Part model, mm, in its own coordinate system. Face numbers are marked on the shaded views. A direction names the side the tool comes from. Round coordinates to 2 decimals unless told otherwise and drop trailing zeros. Order: outer loops, then holes, each group sorted by start corner. A loop starts at its lowest first (then second) coordinate and runs counter-clockwise, first axis right, second up. Notation, with made-up numbers: (-26.75, -31) -> (14.25, -31) arc R28 cw to (14.25, 7) -> close; hole circle Ø3 at (39.25, 54). An arc over 180 degrees is marked (long way). Return JSON: item names as keys, results as strings. Group by question number.
from build123d import *

# Parameters (mm, degrees)
ESQUISSE1_W             = 82.5
ESQUISSE1_H             = 16.543047786
BOSS_EXTRU_1_DEPTH      = 10
CONG_1_R                = 10
ESQUISSE2_W             = 5
ESQUISSE2_H             = 5
ENL_V_MAT_EXTRU_2_DEPTH = 21
ESQUISSE4_W             = 5
ESQUISSE4_H             = 5
ENL_V_MAT_EXTRU_3_DEPTH = 100
ESQUISSE5_R             = 5.960029696
ESQUISSE5_R_2           = 5.029757688
BOSS_EXTRU_4_DEPTH      = 80
ESQUISSE8_R             = 4.979256744
ENL_V_MAT_EXTRU_5_DEPTH = 80
ESQUISSE9_W             = 44.615478915
ESQUISSE9_H             = 9.98536909
BOSS_EXTRU_5_DEPTH      = 10
ESQUISSE10_W            = 10
ESQUISSE10_H            = 10
BOSS_EXTRU_6_DEPTH      = 5
ESQUISSE13_W            = 10
ESQUISSE13_H            = 5
BOSS_EXTRU_7_DEPTH      = 80
ESQUISSE15_R            = 4.979256744
ENL_V_MAT_EXTRU_6_DEPTH = 80


with BuildPart() as part:
    # Esquisse1 → Boss.-Extru.1 (new body)
    with BuildSketch(Plane(origin=(0, 0, 0), x_dir=(1, 0, 0), z_dir=(0, 1, 0))):
        with Locations((-15.683865756, -16.543047786)):
            Rectangle(ESQUISSE1_W, ESQUISSE1_H)
    extrude(amount=BOSS_EXTRU_1_DEPTH)

    # Congé1
    cong_1_edges = [part.edges().sort_by_distance(p)[0] for p in [
        (25.566134244, 5, 24.814571679),
        (-56.933865756, 5, 24.814571679),
    ]]
    fillet(cong_1_edges, radius=CONG_1_R)

    # Esquisse2 → Enlèv. mat.-Extru.2 (cut)
    with BuildSketch(Plane.XY.offset(24.814571679)):
        with Locations((-42.433865756, 5)):
            Rectangle(ESQUISSE2_W, ESQUISSE2_H)
    extrude(amount=-ENL_V_MAT_EXTRU_2_DEPTH, mode=Mode.SUBTRACT)

    # Esquisse4 → Enlèv. mat.-Extru.3 (cut)
    with BuildSketch(Plane.XY.offset(24.814571679)):
        with Locations((11.066134244, 5)):
            Rectangle(ESQUISSE4_W, ESQUISSE4_H)
    extrude(amount=-ENL_V_MAT_EXTRU_3_DEPTH, mode=Mode.SUBTRACT)

    # Esquisse5 → Boss.-Extru.4 (add)
    with BuildSketch(Plane.XY.offset(24.814571679)):
        with Locations((-15.683865756, 5)):
            Circle(ESQUISSE5_R)
        with Locations((-15.683865756, 5)):
            Circle(ESQUISSE5_R_2, mode=Mode.SUBTRACT)
    extrude(amount=-BOSS_EXTRU_4_DEPTH)

    # Esquisse8 → Enlèv. mat.-Extru.5 (cut)
    with BuildSketch(Plane.XY.offset(24.814571679)):
        with Locations((-15.514565948, 5)):
            Circle(ESQUISSE8_R)
    extrude(amount=-ENL_V_MAT_EXTRU_5_DEPTH, mode=Mode.SUBTRACT)

    # Esquisse9 → Boss.-Extru.5 (add)
    with BuildSketch(Plane(origin=(0, 0, 0), x_dir=(1, 0, 0), z_dir=(0, 1, 0))):
        with Locations((-13.028182488, -15.142474607)):
            Rectangle(ESQUISSE9_W, ESQUISSE9_H)
    extrude(amount=BOSS_EXTRU_5_DEPTH)

    # Esquisse10 → Boss.-Extru.6 (add)
    with BuildSketch(Plane(origin=(0, 0, 0), x_dir=(-1, 0, 0), z_dir=(0, -1, 0))):
        with Locations((15.433865756, -19.305846435)):
            Rectangle(ESQUISSE10_W, ESQUISSE10_H)
    extrude(amount=BOSS_EXTRU_6_DEPTH)

    # Esquisse13 → Boss.-Extru.7 (add)
    with BuildSketch(Plane(origin=(0, 0, 14.305846435), x_dir=(-1, 0, 0), z_dir=(0, 0, -1))):
        with Locations((15.433865756, -2.5)):
            Rectangle(ESQUISSE13_W, ESQUISSE13_H)
    extrude(amount=BOSS_EXTRU_7_DEPTH)

    # Esquisse15 → Enlèv. mat.-Extru.6 (cut)
    with BuildSketch(Plane.XY.offset(20.135159152)):
        with Locations((-15.514565948, 5)):
            Circle(ESQUISSE15_R)
    extrude(amount=-ENL_V_MAT_EXTRU_6_DEPTH, mode=Mode.SUBTRACT)


solid = part.part
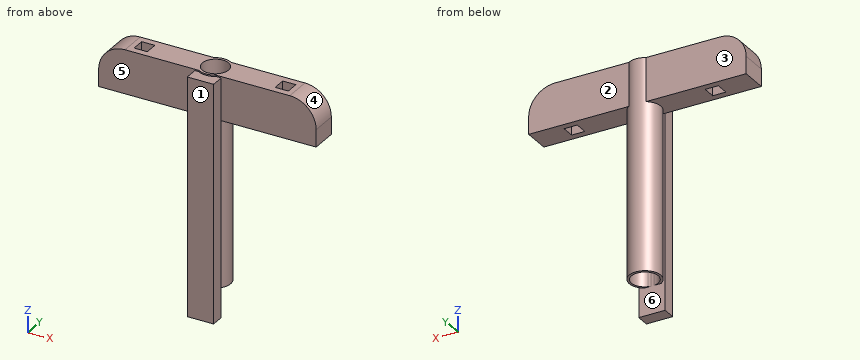
(1) Pin check, flat tips, straight feed: P1, Ø5.5, axis at x = -18, y = 5.5, coming from the -Z side; P2, Ø3, axis at x = -22.5, z = -1.5, coming from the +Y side; P3, Ø1.5, axis at x = -42.5, z = 17, coming from the -Y side. Stop position of each tip, or through.
(2) Saw through at D-D, the plane x = -25. List the corners of the cut face in (y, z), and give its area (3 significant figures).
(3) Saw through at B-B, the plane z = -18. List the corners of the cut face in (x, y), and give its area (3 significant figures).
(4) Saw through at A-A, the plane y = 5. List the corners of the cut face in (x, z), and give its area (3 significant figures).
(5) Mould opens along X. For the marked faces 4, 5 and 6 say: pulls with the +X half, pulls with the -X half, needs draft (parallel to the pull), parting line crosses it, or undercut.
(6) Tool access for the marked faces 1, 2 and 3: list every direction of +Z, -Z, +X, -X, +Y, -Y with a clear straight run to the whole face (end or side of a thin tool).
(7) Probe L1, parallel to X at y = 5, z = -26.5; L2, parallel to X at y = -1, z = -17; L3, parallel to Z at x = -5, y = 4. List the from-to ranges inside material, lowest first. Write a range as [from, to].
(8) Saw through at C-C, the plane z = 16. List the corners of the cut face in (x, y), and give its area (3 significant figures).
Results are:
{
 "1": {"P1": "stops at z = -55.19", "P2": "stops at y = 7.69", "P3": "stops at y = 0"},
 "2": {"outline": "(0, 8.27) -> (10, 8.27) -> (10, 24.81) -> (0, 24.81) -> close", "area": "165 mm^2"},
 "3": {"outline": "(-20.43, -5) -> (-10.43, -5) -> (-10.43, 0) -> (-12.44, 0) arc R5.96 ccw (long way) to (-18.93, 0) -> (-20.43, 0) -> close; hole (-16.23, 0) -> (-15.14, 0) arc R5.03 ccw to (-14.11, 0.22) arc R4.98 ccw to (-14.11, 9.78) arc R5.03 ccw (long way) to start", "area": "76.9 mm^2"},
 "4": {"outline": "(-56.93, 8.27) -> (-44.93, 8.27) -> (-44.93, 24.81) -> (-46.93, 24.81) arc R10 ccw to (-56.93, 14.81) -> close; (-39.93, 8.27) -> (-21.64, 8.27) -> (-21.64, -55.19) -> (-20.71, -55.19) -> (-20.71, 8.27) -> (-20.49, 8.27) -> (-20.49, 24.81) -> (-39.93, 24.81) -> close; (-10.54, -55.19) -> (-9.72, -55.19) -> (-9.72, 8.27) -> (8.57, 8.27) -> (8.57, 10.15) -> (9.28, 10.15) -> (9.28, 20.14) -> (8.57, 20.14) -> (8.57, 24.81) -> (-10.54, 24.81) -> close; (13.57, 8.27) -> (25.57, 8.27) -> (25.57, 14.81) arc R10 ccw to (15.57, 24.81) -> (13.57, 24.81) -> close", "area": "1,110 mm^2"},
 "5": {"face 4": "pulls with the +X half", "face 5": "needs draft", "face 6": "undercut"},
 "6": {"face 1": "+Z, -Z, +X, -X, -Y", "face 2": "+Z, -Z, +X, +Y", "face 3": "+Z, -Z, -X, +Y"},
 "7": {"L1": "x = [-21.64, -20.71], [-10.54, -9.72]", "L2": "x = [-20.43, -10.43]", "L3": "z = [8.27, 24.81]"},
 "8": {"outline": "(-56.86, 0) -> (-20.43, 0) -> (-20.43, -5) -> (-10.43, -5) -> (-10.43, 0) -> (25.5, 0) -> (25.5, 10) -> (-12.44, 10) arc R5.96 ccw to (-18.93, 10) -> (-56.86, 10) -> close; hole (-44.93, 2.5) -> (-39.93, 2.5) -> (-39.93, 7.5) -> (-44.93, 7.5) -> close; hole circle Ø9.96 at (-15.51, 5); hole (-16.23, 10) -> (-15.14, 10) arc R5.03 ccw to start; hole (9.28, 2.5) -> (13.57, 2.5) -> (13.57, 7.5) -> (9.28, 7.5) -> close", "area": "753 mm^2"}
}
